```python
from build123d import *

# Parameters (mm, degrees)
Y_KSEKLIK_EKSTR_ZYON1_DEPTH = 2
Y_KSEKLIK_EKSTR_ZYON2_DEPTH = 3
IZIM5_R                     = 1.55
KES_EKSTR_ZYON1_DEPTH       = 5
IZIM6_R                     = 3.25
KES_EKSTR_ZYON2_DEPTH       = 1.5
KES_EKSTR_ZYON3_DEPTH       = 2


with BuildPart() as part:
    # Çizim1 → Yükseklik-Ekstrüzyon1 (new body)
    with BuildSketch(Plane.XY):
        with BuildLine():
            Line((-41.105081413, 11.299639377), (-8.113863068, 0.378628673))
            ThreePointArc((-8.113863068, 0.378628673), (4.01642262, -10.494132055), (-4.623817667, -24.303802743))
            ThreePointArc((-4.623817667, -24.303802743), (-4.799274482, -24.430880762), (-4.866322935, -24.63688664))
            Line((-4.866322935, -24.63688664), (-4.866322935, -37.083207178))
            ThreePointArc((-4.866322935, -37.083207178), (-4.763810308, -37.330694551), (-4.516322935, -37.433207178))
            Line((-4.516322935, -37.433207178), (18.719678074, -37.433207178))
            ThreePointArc((18.719678074, -37.433207178), (23.009675893, -35.764918267), (25.045514407, -31.636646144))
            Line((25.045514407, -31.636646144), (27.678537645, -1.541052822))
            ThreePointArc((27.678537645, -1.541052822), (27.678537645, -1.480043802), (27.66794354, -1.419961646))
            Line((27.66794354, -1.419961646), (22.642489235, 17.335289151))
            ThreePointArc((22.642489235, 17.335289151), (22.596275233, 17.43788043), (22.519896712, 17.520506249))
            Line((22.519896712, 17.520506249), (-12.9405872, 45.225272639))
            ThreePointArc((-12.9405872, 45.225272639), (-15.548952522, 46.436682119), (-18.424200647, 46.373193573))
            ThreePointArc((-18.424200647, 46.373193573), (-36.179435446, 35.192251208), (-44.076039074, 15.752459901))
            ThreePointArc((-44.076039074, 15.752459901), (-43.356576828, 13.014957214), (-41.105081413, 11.299639377))
        make_face()
    extrude(amount=-Y_KSEKLIK_EKSTR_ZYON1_DEPTH)

    # Çizim4 → Yükseklik-Ekstrüzyon2 (add)
    with BuildSketch(Plane(origin=(0, 0, -2), x_dir=(-1, 0, 0), z_dir=(0, 0, -1))):
        with BuildLine():
            Line((40.146596848, 14.195119879), (28.474092029, 10.331196191))
            Line((28.474092029, 10.331196191), (8.232284194, 3.630594906))
            ThreePointArc((8.232284194, 3.630594906), (7.642809613, 3.577387775), (7.090841177, 3.791027954))
            Line((7.090841177, 3.791027954), (5.755688832, 4.702398932))
            ThreePointArc((5.755688832, 4.702398932), (5.105662961, 4.970115176), (4.402900206, 4.951945686))
            ThreePointArc((4.402900206, 4.951945686), (4.10459824, 4.878061515), (3.807624001, 4.799009418))
            ThreePointArc((3.807624001, 4.799009418), (-6.360722696, -2.664063163), (-8.978039182, -15.002717113))
            ThreePointArc((-8.978039182, -15.002717113), (-8.865317675, -15.645084598), (-8.729007726, -16.282863339))
            ThreePointArc((-8.729007726, -16.282863339), (-8.359304972, -17.008921436), (-7.694222234, -17.479565078))
            Line((-7.694222234, -17.479565078), (-6.567842625, -17.921440305))
            ThreePointArc((-6.567842625, -17.921440305), (-6.142840412, -18.193337265), (-5.853364231, -18.606566472))
            ThreePointArc((-5.853364231, -18.606566472), (-3.610330722, -22.245790214), (-0.468752496, -25.145037533))
            Line((-0.468752496, -25.145037533), (-0.094474949, -25.398000973))
            ThreePointArc((-0.094474949, -25.398000973), (0.169709223, -25.567322514), (0.437224607, -25.73133038))
            Line((0.437224607, -25.73133038), (0.437224607, -34.383207178))
            Line((0.437224607, -34.383207178), (-5.021308607, -34.383207178))
            ThreePointArc((-5.021308607, -34.383207178), (-5.624718884, -33.868281437), (-6.396081315, -33.683207178))
            Line((-6.396081315, -33.683207178), (-6.780735729, -33.683207178))
            Line((-6.780735729, -33.683207178), (-14.98347518, -33.683207178))
            Line((-14.98347518, -33.683207178), (-18.719678074, -33.683207178))
            ThreePointArc((-18.719678074, -33.683207178), (-20.476212614, -33.000128254), (-21.309784289, -31.309812109))
            Line((-21.309784289, -31.309812109), (-21.406910581, -30.199653517))
            ThreePointArc((-21.406910581, -30.199653517), (-21.372380233, -29.76841651), (-21.198254298, -29.37238891))
            Line((-21.198254298, -29.37238891), (-20.618946502, -28.490888179))
            ThreePointArc((-20.618946502, -28.490888179), (-20.391243356, -27.973005932), (-20.346088286, -27.409080615))
            Line((-20.346088286, -27.409080615), (-20.37341709, -27.096710955))
            Line((-20.37341709, -27.096710955), (-22.555546966, -2.154852341))
            ThreePointArc((-22.555546966, -2.154852341), (-22.555546966, -1.92824741), (-22.516197432, -1.705085117))
            Line((-22.516197432, -1.705085117), (-18.284161659, 14.089087411))
            ThreePointArc((-18.284161659, 14.089087411), (-18.112509653, 14.470140733), (-17.828818002, 14.777036632))
            Line((-17.828818002, 14.777036632), (7.059291739, 34.221759043))
            ThreePointArc((7.059291739, 34.221759043), (7.388432983, 34.562743961), (7.61065263, 34.981340548))
            ThreePointArc((7.61065263, 34.981340548), (7.696032795, 35.32414247), (7.70871782, 35.677189239))
            Line((7.70871782, 35.677189239), (7.652642966, 36.498398251))
            ThreePointArc((7.652642966, 36.498398251), (7.762446578, 37.116689055), (8.149262911, 37.611374283))
            Line((8.149262911, 37.611374283), (10.2163345, 39.226347605))
            ThreePointArc((10.2163345, 39.226347605), (10.845026685, 39.490549235), (11.520958616, 39.400147972))
            Line((11.520958616, 39.400147972), (12.009191337, 39.194676987))
            ThreePointArc((12.009191337, 39.194676987), (12.893102324, 39.07645995), (13.715238257, 39.421954389))
            Line((13.715238257, 39.421954389), (16.049677651, 41.245818333))
            ThreePointArc((16.049677651, 41.245818333), (16.583673701, 41.493823423), (17.172307175, 41.480825768))
            ThreePointArc((17.172307175, 41.480825768), (18.108862659, 41.224498821), (19.036372112, 40.937156005))
            ThreePointArc((19.036372112, 40.937156005), (19.943021213, 40.894666775), (20.742308561, 41.32473382))
            Line((20.742308561, 41.32473382), (20.971778793, 41.544527828))
            ThreePointArc((20.971778793, 41.544527828), (21.642700826, 41.88550301), (22.390140455, 41.797557284))
            ThreePointArc((22.390140455, 41.797557284), (35.367714895, 31.255849206), (41.034469252, 15.525847852))
            ThreePointArc((41.034469252, 15.525847852), (40.819457547, 14.7077436), (40.146596848, 14.195119879))
        make_face()
    extrude(amount=Y_KSEKLIK_EKSTR_ZYON2_DEPTH)

    # Çizim5 → Kes-Ekstrüzyon1 (cut)
    with BuildSketch(Plane.XY):
        with Locations((18.588315087, -30.988106158)):
            Circle(IZIM5_R)
        with Locations((8.040668379, -21.065272587)):
            Circle(IZIM5_R)
        with Locations((-22.376194422, 11.828332979)):
            Circle(IZIM5_R)
        with Locations((-10.655916137, 36.555534849)):
            Circle(IZIM5_R)
    extrude(amount=-KES_EKSTR_ZYON1_DEPTH, mode=Mode.SUBTRACT)

    # Çizim6 → Kes-Ekstrüzyon2 (cut)
    with BuildSketch(Plane.XY):
        with Locations((18.588315087, -30.988106158)):
            Circle(IZIM6_R)
        with Locations((8.040668379, -21.065272587)):
            Circle(IZIM6_R)
        with Locations((-22.376194422, 11.828332979)):
            Circle(IZIM6_R)
        with Locations((-10.655916137, 36.555534849)):
            Circle(IZIM6_R)
    extrude(amount=-KES_EKSTR_ZYON2_DEPTH, mode=Mode.SUBTRACT)

    # Çizim7 → Kes-Ekstrüzyon3 (cut)
    with BuildSketch(Plane(origin=(0, 0, -5), x_dir=(-1, 0, 0), z_dir=(0, 0, -1))):
        with BuildLine():
            Line((24.541267724, 38.1096017), (23.517717526, 39.20403478))
            ThreePointArc((23.517717526, 39.20403478), (21.655481578, 40.136777833), (19.634741325, 39.632257115))
            Line((19.634741325, 39.632257115), (16.611199337, 37.567393667))
            ThreePointArc((16.611199337, 37.567393667), (16.488455807, 37.476506841), (16.373005674, 37.376518561))
            Line((16.373005674, 37.376518561), (11.637268483, 32.947499711))
            ThreePointArc((11.637268483, 32.947499711), (11.004872743, 31.563837931), (11.528839766, 30.135586253))
            Line((11.528839766, 30.135586253), (14.814792499, 26.549635137))
            Line((14.814792499, 26.549635137), (27.066921229, 13.449022186))
            ThreePointArc((27.066921229, 13.449022186), (27.732524284, 12.979727648), (28.529940113, 12.814219991))
            Line((28.529940113, 12.814219991), (33.452123381, 12.814639194))
            ThreePointArc((33.452123381, 12.814639194), (34.638107313, 13.059129065), (35.630822107, 13.752562927))
            Line((35.630822107, 13.752562927), (38.266714728, 16.537857285))
            ThreePointArc((38.266714728, 16.537857285), (38.901592885, 17.559574312), (39.084076841, 18.748555205))
            Line((39.084076841, 18.748555205), (38.920753656, 22.041264477))
            ThreePointArc((38.920753656, 22.041264477), (38.764745082, 22.722405414), (38.383934887, 23.308302374))
            Line((38.383934887, 23.308302374), (24.541267724, 38.1096017))
        make_face()
    extrude(amount=-KES_EKSTR_ZYON3_DEPTH, mode=Mode.SUBTRACT)


solid = part.part
```
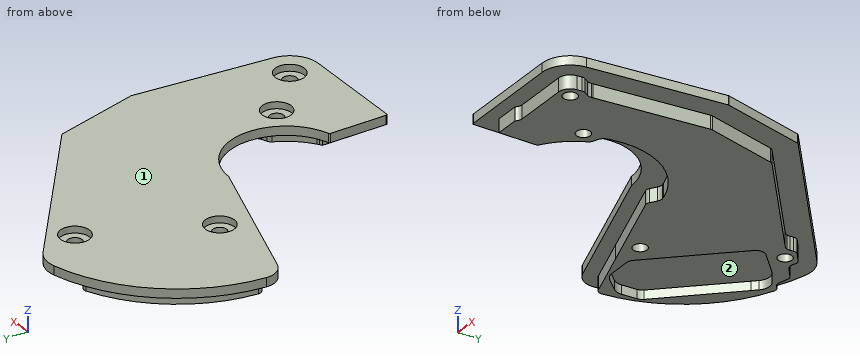
Check sheet for the modelled part. Datum: model origin and axes. Units: mm. Face numbers are marked on the shaded views. A direction names the side the tool comes from. Round coordinates to 2 decimals unless told otherwise and drop trailing zeros. Order: outer loops, then holes, each group sorted by start corner. A loop starts at its lowest first (then second) coordinate and runs counter-clockwise, first axis right, second up.
1) Go/stop test with flat-tipped pins: pin 1 Ø3 at (x, z) = (7, -4) entering from -Y; pin 2 Ø4 at (x, y) = (8.04, -21.07) entering from +Z; pin 3 Ø2 at (x, z) = (-31, -4) entering from +Y. Record where each tip stops, or that it passes through.
2) Tool access check on the marked faces 1 and 2. Record the directions out of +Z, -Z, +X, -X, +Y, -Y that give a thin tool (end or side, any length) a straight path to the whole face; none if there is none.
3) Section check B-B (y = -5.5). Record the boundary of the cut face in (x, z), and give its area (3 significant figures).
4) Section check C-C (x = -31). Record the boundary of the cut face in (y, z), and give its area (3 significant figures).
5) Section check A-A (x = -2). Record the boundary of the cut face in (y, z).
6) Scan lines: line 1 (Y direction, x = 0.5, z = -4.8); line 2 (Y direction, x = -10, z = -0.4); line 3 (Z direction, x = 25, y = -26.5). Record each from-to range of solid material in increasing order.
Result:
1. pin 1: stops at y = -33.94
1. pin 2: stops at z = -1.5
1. pin 3: stops at y = 37.08
2. face 1: +Z, +X, -X, +Y, -Y
2. face 2: -Z
3. outline: (2.18, -2) - (7.85, -2) - (7.85, -5) - (22.26, -5) - (22.26, -2) - (27.33, -2) - (27.33, 0) - (2.18, 0) - close
3. area: 93.6 mm2
4. outline: (7.95, -2) - (11.17, -2) - (11.17, -5) - (12.81, -5) - (12.81, -3) - (31.2, -3) - (31.2, -5) - (36.2, -5) - (36.2, -2) - (40.2, -2) - (40.2, 0) - (7.95, 0) - close
4. area: 103 mm2
5. outline: (-37.43, -2) - (-23.11, -2) - (-23.11, 0) - (-37.43, 0) - close; (-1.42, -2) - (4.19, -2) - (4.19, -5) - (30.27, -5) - (30.27, -2) - (36.68, -2) - (36.68, 0) - (-1.42, 0) - close
6. line 1: y = -34.38 to -25.12, 2.97 to 28.32
6. line 2: y = 1 to 33.37, 39.74 to 42.93
6. line 3: z = -2 to 0
